CAD build for the part. Positions are in the model's coordinates, mm. Give positions to 0.01 mm unless a question says otherwise; leave off trailing zeros. Write each loop counter-clockwise with the first axis right and the second up, starting at its lowest first coordinate (ties: lowest second). Pieces come first, ordered by that corner, then holes. Notation, with made-up numbers: (84, 33) -> (138, 33) arc R28 ccw to (138, 51) -> close; hole circle Ø2 at (32.25, 85). An arc over 180 degrees is marked (long way). Use one line per item in the form item = value. Start each with the question number.
from build123d import *

# Parameters (mm, degrees)
F0_W     = 30.48
F0_H     = 27.94
F1_DEPTH = 12.7
F2_R     = 13.49375
F3_DEPTH = 25.4
F4_W     = 68.546237424
F4_H     = 31.4367190003
F5_DEPTH = 12.7


with BuildPart() as f1:
    # F0 (on Front) → F1 (new body, symmetric)
    with BuildSketch(Plane.XZ):
        Rectangle(F0_W, F0_H)
    extrude(amount=F1_DEPTH, both=True)

    # F2 (on face) → F3 (cut)
    with BuildSketch(Plane.XZ.offset(12.7)):
        Circle(F2_R)
    extrude(amount=-F3_DEPTH, mode=Mode.SUBTRACT)

    # F4 (on Front) → F5 (cut, symmetric)
    with BuildSketch(Plane.XZ):
        with Locations((3.9000464603, 15.7183595002)):
            Rectangle(F4_W, F4_H)
    extrude(amount=F5_DEPTH, both=True, mode=Mode.SUBTRACT)


solid = f1.part
1) Cut at A-A (z = -2.75). Give the cut face in (x, y).
2) Cut at B-B (y = 5.5). Give the cut face in (x, z), and give its area (3 significant figures).
3) Cut at C-C (x = 0). Give the cut face in (y, z), and give its area (3 significant figures).
4) Pin check, flat tips, straight feed: pin 1 (5 mm diameter, centred on x = 5.5, y = 6.5, fed in from +Z); pin 2 (8 mm diameter, centred on x = 11, y = -2.5, fed in from +Z). Stop position of each tip, or through.
5) Cut at D-D (x = -6). Give the cut face in (y, z), and give its area (3 significant figures).
6) Wall check: line 1 along X through (y, z) = (-6.75, -0.25); line 2 along X through (y, z) = (2, -11.75); line 3 along Z through (x, y) = (0, -1.5). Give the ranges that are in metal, low to high. Write a range as from..to.
Final values:
q1.outline = (-15.24, -12.7) -> (-13.21, -12.7) -> (-13.21, 12.7) -> (-15.24, 12.7) -> close; (13.21, -12.7) -> (15.24, -12.7) -> (15.24, 12.7) -> (13.21, 12.7) -> close
q2.outline = (-15.24, -13.97) -> (15.24, -13.97) -> (15.24, 0) -> (13.49, 0) arc R13.49 cw to (-13.49, 0) -> (-15.24, 0) -> close
q2.area = 140 mm^2
q3.outline = (-12.7, -13.97) -> (12.7, -13.97) -> (12.7, -13.49) -> (-12.7, -13.49) -> close
q3.area = 12.1 mm^2
q4.pin_1 = -10.87
q4.pin_2 = 0
q5.outline = (-12.7, -13.97) -> (12.7, -13.97) -> (12.7, -12.09) -> (-12.7, -12.09) -> close
q5.area = 47.8 mm^2
q6.line_1 = -15.24..-13.49, 13.49..15.24
q6.line_2 = -15.24..-6.63, 6.63..15.24
q6.line_3 = -13.97..-13.49
